Design review of the part built by this model. Coordinates are the model's own, in mm. Face numbers are marked on the shaded views. A direction names the side the tool comes from. Round coordinates to 2 decimals unless told otherwise and drop trailing zeros. Loops run counter-clockwise (first coordinate to the right, second up) from the corner with the lowest first, then second, coordinate; pieces in that order, holes last. Notation, with made-up numbers: (23.25, -5.5) - (60.25, -5.5) arc R9 ccw to (60.25, -1.5) - close; hole circle Ø10 at (78, 7.5). An arc over 180 degrees is marked (long way). Return JSON: item names as keys, results as strings. Group by question number.
(1) The part is to be moulded in two halves that separate along Y. For the marked faces 1, 2, 3 and 4, say which applies: pulls with the +Y half, pulls with the -Y half, needs draft (parallel to the pull), parting line crosses it, or undercut.
(2) Wall thickness on L1, parallel to Y at x = 3.9, z = 19; L2, parallel to X at y = 5.5, z = 20.5; L3, parallel to Z at x = 7, y = 0 (3 decimals): over which ranges is each line inside the solid? List them lowest first. Write a range as [from, to].
(3) For the marked faces 5, 6 and 7, list the 3-axis set-ups (+Z, -Z, +X, -X, +Y, -Y) from which the entire face can be reached by the end or side of a thin tool; tool diameter is ignored.
(4) We need section B-B, the plane y = 0. Write out the cut boundary in (x, z) (3 decimals).
(5) We need section C-C, the plane x = 9. Write out the cut boundary in (y, z) (3 decimals), and give its area (3 significant figures).
(6) We need section D-D, the plane y = -5. Give the number of separate pieces and of enclosed holes in the cut face, and give its area (3 significant figures).
(7) We need section A-A, the plane x = 3.5. Write out the cut boundary in (y, z) (3 decimals), and give its area (3 significant figures).
(8) Clearance check with flat-ended pins moving along their axes: pin 1 (2 mm diameter, centred on x = 1.5, y = -0.5, fed in from -Z); pin 2 (3 mm diameter, centred on x = 2.5, y = -4, fed in from +Z); pin 3 (3 mm diameter, centred on y = -1.5, z = 1, fed in from -X); pin 4 (5 mm diameter, centred on y = -1.5, z = 9.5, fed in from +X). State where each tip first meets the part, or that it passes through.
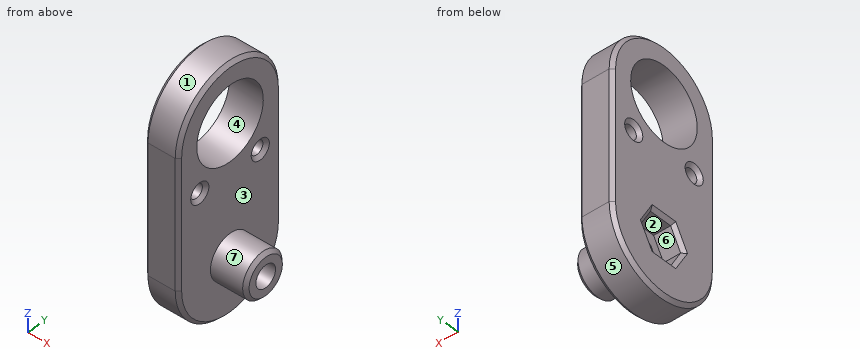
from build123d import *

# Parameters (mm, degrees)
SKETCH1_R           = 1.625
SKETCH1_R_2         = 5.5
SKETCH1_R_3         = 1
BOSS_EXTRUDE1_DEPTH = 5
SKETCH1_3_R         = 3.25
SKETCH1_3_R_2       = 1.625
BOSS_EXTRUDE2_DEPTH = 10.25
CUT_EXTRUDE1_DEPTH  = 3
CHAMFER2_SIZE       = 0.5


with BuildPart() as part:
    # Sketch1 → Boss-Extrude1 (new body)
    with BuildSketch(Plane(origin=(0, 0, 0), x_dir=(0, 0, -1), z_dir=(1, 0, 0))):
        with BuildLine():
            Line((0, -8.5), (-19, -8.5))
            ThreePointArc((-19, -8.5), (-27.5, 0), (-19, 8.5))
            Line((-19, 8.5), (0, 8.5))
            ThreePointArc((0, 8.5), (8.5, 0), (0, -8.5))
        make_face()
        Circle(SKETCH1_R, mode=Mode.SUBTRACT)
        with Locations((-19, 0)):
            Circle(SKETCH1_R_2, mode=Mode.SUBTRACT)
        with Locations((-12.126136458, -5)):
            Circle(SKETCH1_R_3, mode=Mode.SUBTRACT)
        with Locations((-12.126136458, 5)):
            Circle(SKETCH1_R_3, mode=Mode.SUBTRACT)
    extrude(amount=BOSS_EXTRUDE1_DEPTH)

    # Sketch1<3> → Boss-Extrude2 (add)
    with BuildSketch(Plane(origin=(0, 0, 0), x_dir=(0, 0, -1), z_dir=(1, 0, 0))):
        Circle(SKETCH1_3_R)
        Circle(SKETCH1_3_R_2, mode=Mode.SUBTRACT)
    extrude(amount=BOSS_EXTRUDE2_DEPTH)

    # Sketch2 → Cut-Extrude1 (cut)
    with BuildSketch(Plane.ZY):
        Polygon((0, 3.319764048), (-2.875, 1.659882024), (-2.875, -1.659882024), (0, -3.319764048), (2.875, -1.659882024), (2.875, 1.659882024), align=None)
    extrude(amount=-CUT_EXTRUDE1_DEPTH, mode=Mode.SUBTRACT)

    # Chamfer2
    chamfer2_edges = [part.edges().sort_by_distance(p)[0] for p in [
        (0, 5, 13.126136458),
        (0, -5, 13.126136458),
        (0, 0, -8.5),
        (0, -8.5, 9.5),
        (0, 0, 27.5),
        (0, 8.5, 9.5),
        (5, 8.5, 9.5),
        (5, 0, 27.5),
        (5, -8.5, 9.5),
        (5, 0, -8.5),
        (10.25, 0, 3.25),
        (5, -5, 13.126136458),
        (5, 5, 13.126136458),
        (0, -2.489823036, -1.4375),
        (0, -2.489823036, 1.4375),
        (0, 0, 2.875),
        (0, 2.489823036, 1.4375),
        (0, 2.489823036, -1.4375),
        (0, 0, -2.875),
    ]]
    chamfer(chamfer2_edges, length=CHAMFER2_SIZE)


solid = part.part
Solutions:
{
 "1": {"face 1": "parting line crosses it", "face 2": "undercut", "face 3": "needs draft", "face 4": "undercut"},
 "2": {"L1": "[-8.5, -5.5], [5.5, 8.5]", "L2": "[0, 5]", "L3": "[-3.25, -1.625], [1.625, 3.25]"},
 "3": {"face 5": "-Z, +X, -X", "face 6": "-X", "face 7": "+X"},
 "4": {"outline": "(0, -8) - (0.5, -8.5) - (4.5, -8.5) - (5, -8) - (5, -3.25) - (9.75, -3.25) - (10.25, -2.75) - (10.25, -1.625) - (3, -1.625) - (3, -2.875) - (0.5, -2.875) - (0, -3.375) - close; (0, 3.375) - (0.5, 2.875) - (3, 2.875) - (3, 1.625) - (10.25, 1.625) - (10.25, 2.75) - (9.75, 3.25) - (5, 3.25) - (5, 13.5) - (0, 13.5) - close; (0, 24.5) - (5, 24.5) - (5, 27) - (4.5, 27.5) - (0.5, 27.5) - (0, 27) - close"},
 "5": {"outline": "circle Ø6.5 at (0, 0); hole circle Ø3.25 at (0, 0)", "area": "24.9 mm^2"},
 "6": {"separate pieces": "3", "enclosed holes": "0", "area": "130 mm^2"},
 "7": {"outline": "(-8.5, 0) arc R8.5 ccw to (8.5, 0) - (8.5, 19) arc R8.5 ccw to (-8.5, 19) - close; hole circle Ø2 at (-5, 12.126); hole circle Ø11 at (0, 19); hole circle Ø3.25 at (0, 0); hole circle Ø2 at (5, 12.126)", "area": "440 mm^2"},
 "8": {"pin 1": "z = -8.5", "pin 2": "z = 27.12", "pin 3": "x = 0.08", "pin 4": "x = 5"}
}
